Source: three-view drawing plus pictorial views. Frame: mm from the lowest corner of the part. Round coordinates to 2 decimals unless told otherwise and drop trailing zeros. Order: outer loops, then holes, each group sorted by start corner. A loop starts at its lowest first (then second) coordinate and runs counter-clockwise, first axis right, second up. Notation, with made-up numbers: (-35, 9.5) -> (7, 9.5) arc R14 cw to (7, 34.5) -> close; hole circle Ø2 at (-23.75, 70). An arc over 180 degrees is marked (long way). Use a Markdown table: item, result.
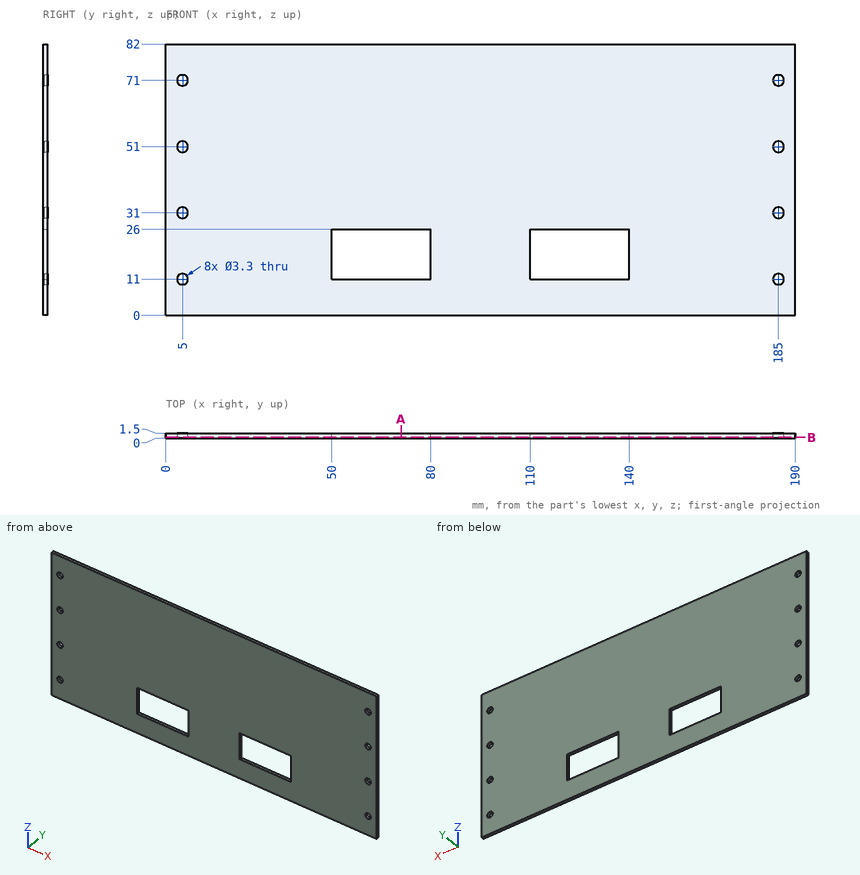
1) Pin query (flat end, axial travel): pin 1 Ø8 at (x, z) = (61, 45) entering from -Y. Return the tip coordinate at first contact, or that it passes through.
Results found:
| item | result |
|---|---|
| pin 1 | stops at y = 0 |
2) Line query: L1, parallel to Z at x = 5, y = 0.4; L2, parallel to X at y = 0.15, z = 19.5; L3, parallel to Z at x = 112, y = 0.95. Output: solid intervals per line, ascending. Write a range as [from, to].
Results found:
| item | result |
|---|---|
| L1 | z = [0, 9.35], [12.65, 29.35], [32.65, 49.35], [52.65, 69.35], [72.65, 82] |
| L2 | x = [0, 50], [80, 110], [140, 190] |
| L3 | z = [0, 11], [26, 82] |
3) Cut plane A-A on x = 71. Return loops of the section in (y, z), and give its area (4 significant figures).
Results found:
| item | result |
|---|---|
| outline | (0, 0) -> (1.5, 0) -> (1.5, 11) -> (0, 11) -> close; (0, 26) -> (1.5, 26) -> (1.5, 82) -> (0, 82) -> close |
| area | 100.5 mm² |
4) Cut plane B-B on y = 0.35. Count the separate pieces of the cut face and the enclosed holes in it, and give its area (3 significant figures).
Results found:
| item | result |
|---|---|
| separate pieces | 1 |
| enclosed holes | 10 |
| area | 14,600 mm² |
